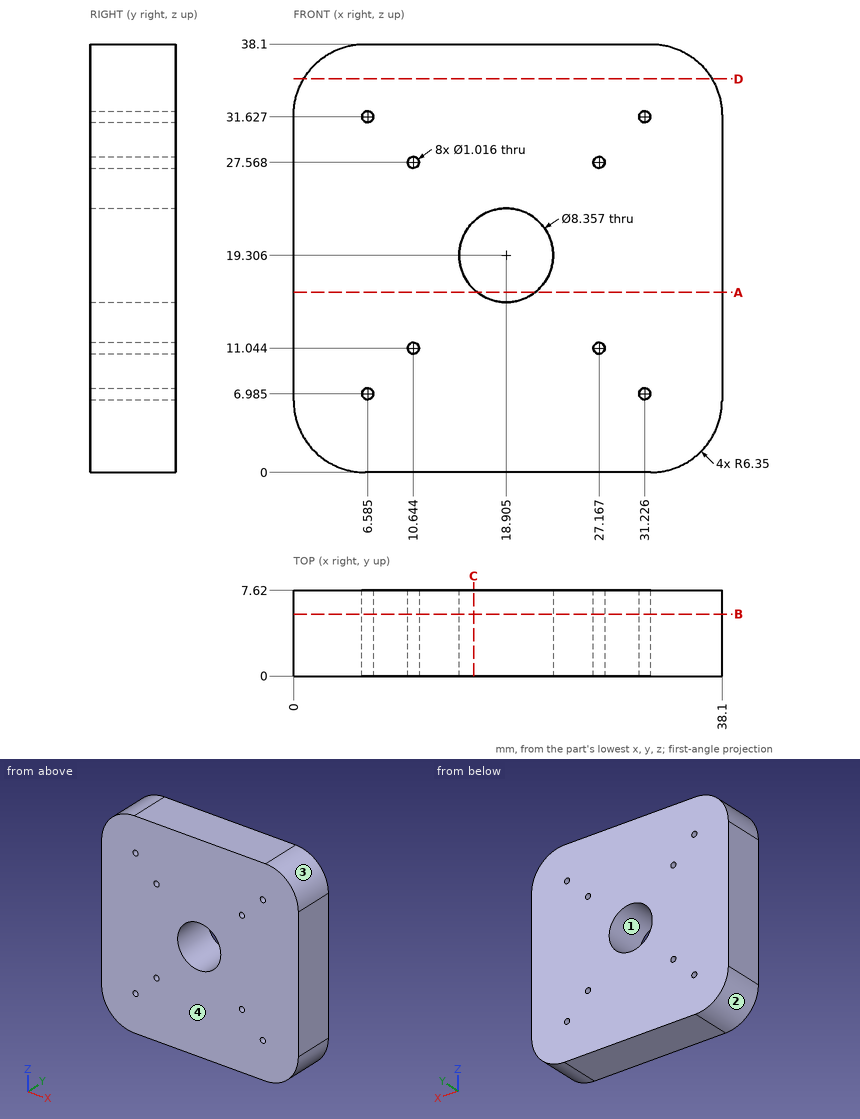
Can you work these out from the drawing? Everything is in mm from the part's minimum corner. Give positions to 0.01 mm unless a question says otherwise; leave off trailing zeros. Order: outer loops, then holes, each group sorted by start corner. A loop starts at its lowest first (then second) coordinate and runs counter-clockwise, first axis right, second up. Notation, with made-up numbers: M 20,55 L 25,55 A30 cw 25,85 Z; hole C 10,15.25 d2. An arc over 180 degrees is marked long. Use a Markdown table: item, result. Add a question column.
Item 1: Suppose I cut it at C-C (x = 16). List the corners of the cut face in (y, z) for me.
Item 2: Suppose I cut it at A-A (z = 16). List the corners of the cut face in (x, y) for me, then the cut area to 3 significant figures.
Item 3: Suppose I cut it at D-D (z = 35). List the corners of the cut face in (x, y) for me (1 decimal).
Item 4: Suppose I cut it at B-B (y = 5.5). Count the separate pieces of the cut face and the enclosed holes in it, then the cut area to 3 significant figures.
Item 5: If I drill on L1, parallel to Z at x = 11, y = 6.5 (1 decimal); L2, parallel to Z at x = 27, y = 1 (1 decimal); L3, parallel to Z at x = 19, y = 2, over which ranges is the centre line in solid material (lowest first)? Write a range as [from, to].
Item 6: We'd pull the mould along Z, two halves only. Please class the marked faces 1, 2, 3 and 4: +Z half, -Z half, draft (parallel to the pull), parting line (faces both ways), or undercut.
Answer sheet:
| question | item | result |
|---|---|---|
| 1 | outline | M 0,0 L 7.62,0 L 7.62,16.3 L 0,16.3 Z; M 0,22.31 L 7.62,22.31 L 7.62,38.1 L 0,38.1 Z |
| 2 | outline | M 0,0 L 16.35,0 L 16.35,7.62 L 0,7.62 Z; M 21.46,0 L 38.1,0 L 38.1,7.62 L 21.46,7.62 Z |
| 2 | area | 251 mm² |
| 3 | outline | M 0.9,0 L 37.2,0 L 37.2,7.6 L 0.9,7.6 Z |
| 4 | separate pieces | 1 |
| 4 | enclosed holes | 9 |
| 4 | area | 1,360 mm² |
| 5 | L1 | z = [0, 10.7], [11.4, 27.2], [27.9, 38.1] |
| 5 | L2 | z = [0, 10.6], [11.5, 27.1], [28, 38.1] |
| 5 | L3 | z = [0, 15.13], [23.48, 38.1] |
| 6 | face 1 | undercut |
| 6 | face 2 | -Z half |
| 6 | face 3 | +Z half |
| 6 | face 4 | draft |
